The listing builds one solid part. Answer for the finished solid, in the listing's coordinates (mm). Give positions to 0.01 mm unless a question says otherwise; leave off trailing zeros. Order: outer loops, then holes, each group sorted by start corner. A loop starts at its lowest first (then second) coordinate and runs counter-clockwise, first axis right, second up. Notation, with made-up numbers: M 73.25,54.5 L 89.25,54.5 A22 cw 89.25,75.5 Z; hole C 73.25,-7.75 d5. An arc over 180 degrees is marked long. Answer as a JSON object with one key per item and string values. Group by question number.
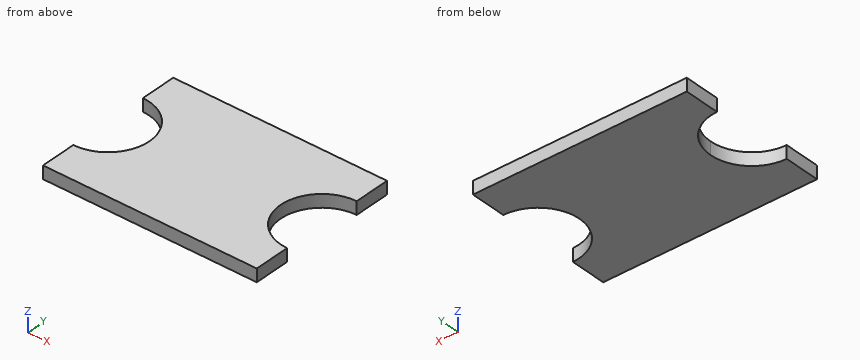
```python
from build123d import *

# Parameters (mm, degrees)
F0_W     = 20
F0_H     = 14.4
F1_DEPTH = 1.2
F3_DEPTH = 25.4


with BuildPart() as f1:
    # F0 (on Top) → F1 (new body)
    with BuildSketch(Plane.XY):
        with Locations((-3.4372447997, -7.5929352783)):
            Rectangle(F0_W, F0_H)
    extrude(amount=F1_DEPTH)

    # F2 (on face) → F3 (cut)
    with BuildSketch(Plane.XY.offset(1.2)):
        with BuildLine():
            ThreePointArc((-13.4372447997, -11.4429352783), (-10.7148836922, -10.3152963859), (-9.5872447997, -7.5929352783))
            ThreePointArc((-9.5872447997, -7.5929352783), (-10.7148836922, -4.8705741708), (-13.4372447997, -3.7429352783))
            Line((-13.4372447997, -3.7429352783), (-13.4372447997, -11.4429352783))
        make_face()
        with BuildLine():
            Line((6.5627552003, -11.4429352783), (6.5627552003, -3.7429352783))
            ThreePointArc((6.5627552003, -3.7429352783), (2.7127552003, -7.5929352783), (6.5627552003, -11.4429352783))
        make_face()
    extrude(amount=-F3_DEPTH, mode=Mode.SUBTRACT)


solid = f1.part
```
Item 1: Consider probe 1 along Y at (x, z) = (4, 0.4); probe 2 along X at (y, z) = (-4.5, 1.05); probe 3 along Y at (x, z) = (3.75, 1.15). Determine where each line is inside the solid, lowest interval first. Write a range as from..to.
Item 2: Section A-A (z = 0.65) is taken. Determine the outline of the cut face in (x, y).
Item 3: Section B-B (x = -10.25) is taken. Determine the outline of the cut face in (y, z), and give its area (3 significant figures).
Item 4: Section D-D (y = -6) is taken. Determine the outline of the cut face in (x, z).
Item 5: Section C-C (y = -10) is taken. Determine the outline of the cut face in (x, z), and give its area (3 significant figures).
Values found:
{
 "1": {"probe 1": "y = -14.79..-10.47, -4.72..-0.39", "probe 2": "x = -11.14..4.27", "probe 3": "y = -14.79..-10.22, -4.96..-0.39"},
 "2": {"outline": "M -13.44,-14.79 L 6.56,-14.79 L 6.56,-11.44 A3.85 cw 6.56,-3.74 L 6.56,-0.39 L -13.44,-0.39 L -13.44,-3.74 A3.85 cw -13.44,-11.44 Z"},
 "3": {"outline": "M -14.79,0 L -9.75,0 L -9.75,1.2 L -14.79,1.2 Z; M -5.43,0 L -0.39,0 L -0.39,1.2 L -5.43,1.2 Z", "area": "12.1 mm^2"},
 "4": {"outline": "M -9.93,0 L 3.06,0 L 3.06,1.2 L -9.93,1.2 Z"},
 "5": {"outline": "M -10.43,0 L 3.56,0 L 3.56,1.2 L -10.43,1.2 Z", "area": "16.8 mm^2"}
}
